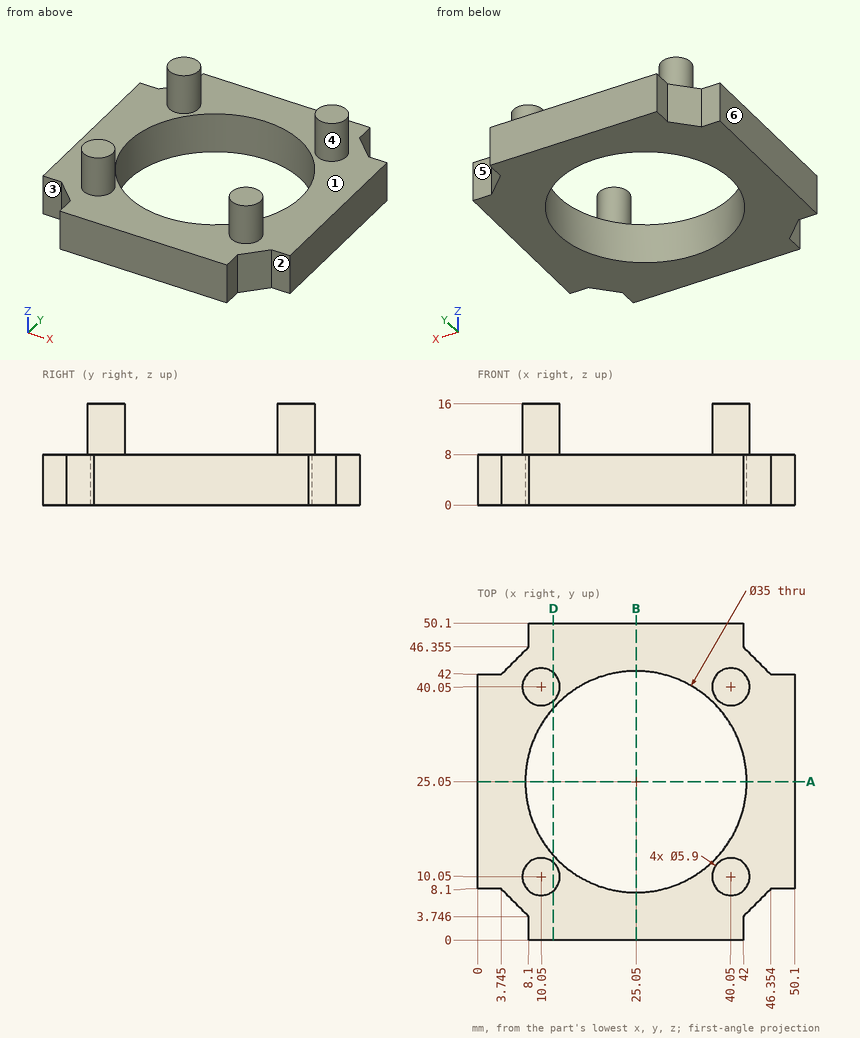
Job drawing, mm, ordinate dimensions from the low corner. One solid piece. A direction names the side the tool comes from. Give positions to 0.01 mm unless a question says otherwise; leave off trailing zeros. Write each loop counter-clockwise with the first axis right and the second up, starting at its lowest first coordinate (ties: lowest second). Pieces come first, ordered by that corner, then holes. Notation, with made-up numbers: (37, -9) - (64, -9) arc R21 cw to (64, 17) - close; hole circle Ø9 at (-38, 77.25). An arc over 180 degrees is marked (long way). Answer as CSV lines item,"result".
1. Drill centre lines: L1, parallel to Y at x = 25.05, z = 6.25; L2, parallel to Z at x = 6, y = 18.5; L3, parallel to X at y = 22, z = 2.75. Where is each one in solid material? Low to high. Write a range as [from, to].
Responses:
L1,"y = [0, 7.55], [42.55, 50.1]"
L2,"z = [0, 8]"
L3,"x = [0, 7.82], [42.28, 50.1]"
2. Two-plate mould, pull along X, no slides. Class the marked faces 4, 5 and 6: +X half, -X half, draft (parallel to the pull), parting line (faces both ways), or undercut.
Responses:
face 4,"undercut"
face 5,"draft"
face 6,"-X half"
3. Pin check, flat tips, straight feed: pin 1 (1.1 mm diameter, centred on x = 47.5, z = 2.5, fed in from +Y); pin 2 (1.9 mm diameter, centred on x = 48.5, z = 4.5, fed in from -Y); pin 3 (4 mm diameter, centred on x = 2.5, z = 4.5, fed in from -Y) (1 decimal). Stop position of each tip, or through.
Responses:
pin 1,"stops at y = 42"
pin 2,"stops at y = 8.1"
pin 3,"stops at y = 7.3"
4. 3-axis set-ups, long thin cutter, end or side, ignore diameter. For the marked faces 1, 2 and 3: which of +Z, -Z, +X, -X, +Y, -Y reach the whole face in a straight line?
Responses:
face 1,"+Z"
face 2,"+Z, -Z, +X, -Y"
face 3,"+Z, -Z, -X, -Y"
5. Band-saw the part on A-A (y = 25.05). Write the cut outline in (x, z).
Responses:
outline,"(0, 0) - (7.55, 0) - (7.55, 8) - (0, 8) - close; (42.55, 0) - (50.1, 0) - (50.1, 8) - (42.55, 8) - close"
6. Band-saw the part on D-D (x = 12). Write the cut outline in (y, z), and give its area (3 significant figures).
Responses:
outline,"(0, 0) - (13.39, 0) - (13.39, 8) - (12.26, 8) - (12.26, 16) - (7.84, 16) - (7.84, 8) - (0, 8) - close; (36.71, 0) - (50.1, 0) - (50.1, 8) - (42.26, 8) - (42.26, 16) - (37.84, 16) - (37.84, 8) - (36.71, 8) - close"
area,"285 mm2"
